Part model, mm, in its own coordinate system. Face numbers are marked on the shaded views. A direction names the side the tool comes from. Round coordinates to 2 decimals unless told otherwise and drop trailing zeros. Loops run counter-clockwise (first coordinate to the right, second up) from the corner with the lowest first, then second, coordinate; pieces in that order, holes last. Notation, with made-up numbers: (87.5, 67.5) -> (104.5, 67.5) arc R23 ccw to (104.5, 81.5) -> close; hole circle Ø7 at (-40, -32.5). An arc over 180 degrees is marked (long way). Answer as a JSON object with one key per item and string values. Group by question number.
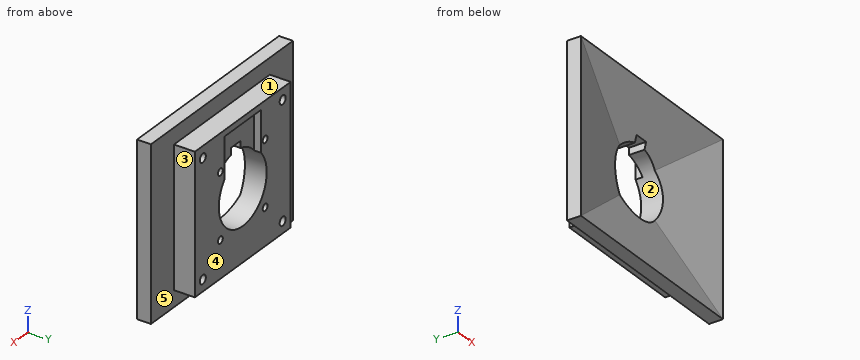
from build123d import *

# Parameters (mm, degrees)
SKETCH1_W           = 60
SKETCH1_H           = 60
BOSS_EXTRUDE1_DEPTH = 15
SKETCH10_W          = 15
SKETCH10_H          = 15
CUT_EXTRUDE4_DEPTH  = 8
SKETCH9_W           = 88.892246252
SKETCH9_H           = 74
SKETCH9_W_2         = 60
SKETCH9_H_2         = 60
BOSS_EXTRUDE4_DEPTH = 6
SKETCH2_R           = 15
CUT_EXTRUDE5_DEPTH  = 60.744940206
SKETCH11_R          = 1.5
CUT_EXTRUDE6_DEPTH  = 6
SKETCH12_W          = 23
SKETCH12_H          = 10.738639716
CUT_EXTRUDE7_DEPTH  = 3
SKETCH13_W          = 23
SKETCH13_H          = 7
CUT_EXTRUDE8_DEPTH  = 3
SKETCH14_R          = 1.875
CUT_EXTRUDE9_DEPTH  = 5
SKETCH15_W          = 6
SKETCH15_H          = 8
CUT_EXTRUDE10_DEPTH = 60.063168554


with BuildPart() as part:
    # Sketch1 → Boss-Extrude1 (new body)
    with BuildSketch(Plane(origin=(0, 0, 0), x_dir=(1, 0, 0), z_dir=(0, 1, 0))):
        Rectangle(SKETCH1_W, SKETCH1_H)
    extrude(amount=BOSS_EXTRUDE1_DEPTH)

    # Sketch10 → Cut-Extrude4 (cut)
    with BuildSketch(Plane(origin=(0, 15, 0), x_dir=(1, 0, 0), z_dir=(0, 1, 0))):
        Rectangle(SKETCH10_W, SKETCH10_H)
    extrude(amount=-CUT_EXTRUDE4_DEPTH, mode=Mode.SUBTRACT)

    # Sketch9 → Boss-Extrude4 (add)
    with BuildSketch(Plane.XZ):
        Rectangle(SKETCH9_W, SKETCH9_H)
        Rectangle(SKETCH9_W_2, SKETCH9_H_2, mode=Mode.SUBTRACT)
    extrude(amount=-BOSS_EXTRUDE4_DEPTH)

    # Cut-Loft2: read off the stored shape, not the designer's step
    # Cut-Loft2: loft between two sections, ruled curve by curve
    cut_loft2_from = [
        Edge.make_line((-7.5, 7, -7.5), (7.5, 7, -7.5)),
        Edge.make_line((7.5, 7, -7.5), (7.5, 7, 7.5)),
        Edge.make_line((-7.5, 7, 7.5), (-7.5, 7, -7.5)),
        Edge.make_line((7.5, 7, 7.5), (-7.5, 7, 7.5)),
    ]
    cut_loft2_to = [
        Edge.make_line((-44.446123126, 0, -37), (44.446123126, 0, -37)),
        Edge.make_line((44.446123126, 0, -37), (44.446123126, 0, 37)),
        Edge.make_line((-44.446123126, 0, 37), (-44.446123126, 0, -37)),
        Edge.make_line((44.446123126, 0, 37), (-44.446123126, 0, 37)),
    ]
    cut_loft2 = Solid(Shell([*[Face.make_surface_from_curves(cut_loft2_from[k], cut_loft2_to[k]) for k in range(4)], Face(Wire(cut_loft2_from)), Face(Wire(cut_loft2_to))]))
    add(cut_loft2, mode=Mode.SUBTRACT)

    # Sketch2 → Cut-Extrude5 (cut, through all)
    with BuildSketch(Plane(origin=(0, 15, 0), x_dir=(1, 0, 0), z_dir=(0, 1, 0))):
        with Locations(Location((0, 0, 0), (0, 0, 270))):
            Circle(SKETCH2_R)
    extrude(amount=-CUT_EXTRUDE5_DEPTH, mode=Mode.SUBTRACT)

    # Sketch11 → Cut-Extrude6 (cut)
    with BuildSketch(Plane(origin=(0, 15, 0), x_dir=(1, 0, 0), z_dir=(0, 1, 0))):
        with Locations(Location((-14, 14, 0), (0, 0, 270))):
            Circle(SKETCH11_R)
        with Locations(Location((14, 14, 0), (0, 0, 270))):
            Circle(SKETCH11_R)
        with Locations(Location((14, -14, 0), (0, 0, 270))):
            Circle(SKETCH11_R)
        with Locations(Location((-14, -14, 0), (0, 0, 270))):
            Circle(SKETCH11_R)
    extrude(amount=-CUT_EXTRUDE6_DEPTH, mode=Mode.SUBTRACT)

    # Sketch12 → Cut-Extrude7 (cut)
    with BuildSketch(Plane(origin=(0, 15, 0), x_dir=(1, 0, 0), z_dir=(0, 1, 0))):
        with Locations((0, -15)):
            Rectangle(SKETCH12_W, SKETCH12_H)
    extrude(amount=-CUT_EXTRUDE7_DEPTH, mode=Mode.SUBTRACT)

    # Sketch13 → Cut-Extrude8 (cut)
    with BuildSketch(Plane(origin=(0, 15, 0), x_dir=(1, 0, 0), z_dir=(0, 1, 0))):
        with Locations((0, -23.869319858)):
            Rectangle(SKETCH13_W, SKETCH13_H)
    extrude(amount=-CUT_EXTRUDE8_DEPTH, mode=Mode.SUBTRACT)

    # Sketch14 → Cut-Extrude9 (cut)
    with BuildSketch(Plane(origin=(0, 15, 0), x_dir=(1, 0, 0), z_dir=(0, 1, 0))):
        with Locations(Location((-25, 25, 0), (0, 0, 270))):
            Circle(SKETCH14_R)
        with Locations(Location((25, 25, 0), (0, 0, 270))):
            Circle(SKETCH14_R)
        with Locations(Location((25, -25, 0), (0, 0, 270))):
            Circle(SKETCH14_R)
        with Locations(Location((-25, -25, 0), (0, 0, 270))):
            Circle(SKETCH14_R)
    extrude(amount=-CUT_EXTRUDE9_DEPTH, mode=Mode.SUBTRACT)

    # Sketch15 → Cut-Extrude10 (cut, through all)
    with BuildSketch(Plane(origin=(0, 12, 0), x_dir=(1, 0, 0), z_dir=(0, 1, 0))):
        with Locations((0, -13.684659929)):
            Rectangle(SKETCH15_W, SKETCH15_H)
    extrude(amount=-CUT_EXTRUDE10_DEPTH, mode=Mode.SUBTRACT)


solid = part.part
Item 1: Two-plate mould, pull along X, no slides. Class the marked faces 1, 2 and 3: pulls with the +X half, pulls with the -X half, needs draft (parallel to the pull), parting line crosses it, or undercut.
Item 2: Drop flat-ended pins along their axis: pin 1 Ø2 at (y, z) = (10.5, -4.5) entering from -X; pin 2 Ø1.8 at (x, z) = (14, 14) entering from +Y; pin 3 Ø3.5 at (x, z) = (-14, 14) entering from +Y; pin 4 Ø5.5 at (x, z) = (-3.5, 17.5) entering from +Y. Give the stop position or say it passes through.
Item 3: Drill centre lines: line 1 (X direction, y = 11.45, z = -25) (3 decimals); line 2 (X direction, y = 12.45, z = 14); line 3 (X direction, y = 11.5, z = -13). Where is each one in solid material? Low to high.
Item 4: Band-saw the part on B-B, the plane y = 13.5. Count the separate pieces of the cut face and the enclosed holes in it, plus the area to 3 significant figures.
Item 5: Which spindle directions (+Z, -Z, +X, -X, +Y, -Y) get a long thin tool onto all of the face, cutting with end or side? Do the marked faces 4 and 5. Say none if no direction does.
Item 6: Band-saw the part on A-A, the plane y = 8. List the corners of the cut face in (x, z).
Entries:
{
 "1": {"face 1": "needs draft", "face 2": "undercut", "face 3": "pulls with the +X half"},
 "2": {"pin 1": "x = -30", "pin 2": "y = 9", "pin 3": "y = 15", "pin 4": "y = 12"},
 "3": {"line 1": "-30 to -26.875, -23.125 to 23.125, 26.875 to 30", "line 2": "-30 to -15.5, -12.5 to -11.5, 11.5 to 12.5, 15.5 to 30", "line 3": "-30 to -15.12, -12.88 to -7.48, 7.48 to 12.88, 15.12 to 30"},
 "4": {"separate pieces": "1", "enclosed holes": "9", "area": "2,500 mm²"},
 "5": {"face 4": "+Z, -Z, +X, -X, +Y", "face 5": "+Y"},
 "6": {"outline": "(-30, -30) -> (30, -30) -> (30, 30) -> (-30, 30) -> close; hole (-3, 14.7) arc R15 ccw (long way) to (3, 14.7) -> (3, 17.68) -> (-3, 17.68) -> close"}
}
